Design review of the part built by this model. Coordinates are the model's own, in mm. A direction names the side the tool comes from. Coordinates: 2 decimals unless noted, no trailing zeros. Order: outer loops, then holes, each group sorted by start corner. A loop starts at its lowest first (then second) coordinate and runs counter-clockwise, first axis right, second up. Notation, with made-up numbers: M -39.75,18.25 L -19.75,18.25 A29 ccw -19.75,48.25 Z; hole C -31,-12.5 d11. An arc over 180 degrees is marked long. Use CSV: the item, a comma, the result in double quotes.
```python
from build123d import *

# Parameters (mm, degrees)
SKETCH_1_R          = 1.75
SKETCH_1_R_2        = 3
EXTRUDE_1_DEPTH     = 3
SKETCH_3_R          = 1.525
CUT_EXTRUDE_2_DEPTH = 10
SKETCH_5_R          = 1.55
CUT_EXTRUDE_3_DEPTH = 10


with BuildPart() as part:
    # 草图1 → 凸台-拉伸1 (new body)
    with BuildSketch(Plane.XY):
        Polygon((65, -25), (65, 75.163369284), (39.840227583, 104.667600302), (-39.840227583, 104.667600302), (-65, 75.163369284), (-65, -25), (-65, -35.332399698), (65, -35.332399698), align=None)
        with Locations((49.25, -15.332399698)):
            Circle(SKETCH_1_R, mode=Mode.SUBTRACT)
        with Locations((25.25, -15.332399698)):
            Circle(SKETCH_1_R, mode=Mode.SUBTRACT)
        with Locations((25.25, 15)):
            Circle(SKETCH_1_R, mode=Mode.SUBTRACT)
        with Locations((49.25, 15)):
            Circle(SKETCH_1_R, mode=Mode.SUBTRACT)
        with Locations(Location((-49.25, 15, 0), (0, 0, 180))):
            Circle(SKETCH_1_R, mode=Mode.SUBTRACT)
        with Locations(Location((-25.25, 15, 0), (0, 0, 180))):
            Circle(SKETCH_1_R, mode=Mode.SUBTRACT)
        with Locations(Location((-25.25, -15.332399698, 0), (0, 0, 180))):
            Circle(SKETCH_1_R, mode=Mode.SUBTRACT)
        with Locations(Location((-49.25, -15.332399698, 0), (0, 0, 180))):
            Circle(SKETCH_1_R, mode=Mode.SUBTRACT)
        with Locations((-17.5, 94.667600302)):
            Circle(SKETCH_1_R_2, mode=Mode.SUBTRACT)
        with Locations(Location((17.5, 94.667600302, 0), (0, 0, 180))):
            Circle(SKETCH_1_R_2, mode=Mode.SUBTRACT)
        with Locations((-17.5, 49.667600302)):
            Circle(SKETCH_1_R_2, mode=Mode.SUBTRACT)
        with Locations(Location((17.5, 49.667600302, 0), (0, 0, 180))):
            Circle(SKETCH_1_R_2, mode=Mode.SUBTRACT)
        with BuildLine():
            Line((-10, 39.667600302), (10, 39.667600302))
            ThreePointArc((10, 39.667600302), (11.5, 38.167600302), (10, 36.667600302))
            Line((10, 36.667600302), (-10, 36.667600302))
            ThreePointArc((-10, 36.667600302), (-11.5, 38.167600302), (-10, 39.667600302))
        make_face(mode=Mode.SUBTRACT)
        with BuildLine():
            Line((-10, -18.332399698), (10, -18.332399698))
            ThreePointArc((10, -18.332399698), (11.5, -19.832399698), (10, -21.332399698))
            Line((10, -21.332399698), (-10, -21.332399698))
            ThreePointArc((-10, -21.332399698), (-11.5, -19.832399698), (-10, -18.332399698))
        make_face(mode=Mode.SUBTRACT)
    extrude(amount=EXTRUDE_1_DEPTH)

    # 草图3 → 切除-拉伸2 (cut)
    with BuildSketch(Plane(origin=(0, 0, 0), x_dir=(-1, 0, 0), z_dir=(0, 0, -1))):
        with Locations((0, -25.832399698)):
            Circle(SKETCH_3_R)
        with BuildLine():
            Line((-18.52, -27.332399698), (-18.52, -24.332399698))
            ThreePointArc((-18.52, -24.332399698), (-17, -22.812399698), (-15.48, -24.332399698))
            Line((-15.48, -24.332399698), (-15.48, -27.332399698))
            ThreePointArc((-15.48, -27.332399698), (-17, -28.852399698), (-18.52, -27.332399698))
        make_face()
        with BuildLine():
            Line((18.52, -27.332399698), (18.52, -24.332399698))
            ThreePointArc((18.52, -24.332399698), (17, -22.812399698), (15.48, -24.332399698))
            Line((15.48, -24.332399698), (15.48, -27.332399698))
            ThreePointArc((15.48, -27.332399698), (17, -28.852399698), (18.52, -27.332399698))
        make_face()
    extrude(amount=-CUT_EXTRUDE_2_DEPTH, mode=Mode.SUBTRACT)

    # 草图5 → 切除-拉伸3 (cut)
    with BuildSketch(Plane.XY.offset(3)):
        with Locations((-47.5, 49.667600302)):
            Circle(SKETCH_5_R)
        with Locations((47.5, 49.667600302)):
            Circle(SKETCH_5_R)
        with Locations((-47.5, -25.332399698)):
            Circle(SKETCH_5_R)
        with Locations((47.5, -25.332399698)):
            Circle(SKETCH_5_R)
    extrude(amount=-CUT_EXTRUDE_3_DEPTH, mode=Mode.SUBTRACT)


solid = part.part
```
(1) Add section A-A on y = 15. State the section outline as (x, z) points.
The answers:
outline,"M -65,0 L -51,0 L -51,3 L -65,3 Z; M -47.5,0 L -27,0 L -27,3 L -47.5,3 Z; M -23.5,0 L 23.5,0 L 23.5,3 L -23.5,3 Z; M 27,0 L 47.5,0 L 47.5,3 L 27,3 Z; M 51,0 L 65,0 L 65,3 L 51,3 Z"
(2) Add section C-C on z = 2.2. Give the number of separate pieces and of enclosed holes in the cut face, and give its area (3 significant figures).
The answers:
separate pieces,"1"
enclosed holes,"21"
area,"17,100 mm2"
(3) For faces 4 (the face through (-15.48, -26, 1)), 5 (the face through (65, 19, 1)), list the 3-axis set-ups (+Z, -Z, +X, -X, +Y, -Y) from which the entire face can be reached by the end or side of a thin tool; tool diameter is ignored.
The answers:
face 4,"+Z, -Z"
face 5,"+Z, -Z, +X, +Y, -Y"
(4) Wall thickness on probe 1 along Y at (x, z) = (-25.5, 0.8); probe 2 along Y at (x, z) = (10, 1.1); probe 3 along Y at (x, z) = (17.5, 1.05): over which ranges is each line inside the solid? List them lowest first.
The answers:
probe 1,"y = -35.33 to -17.06, -13.6 to 13.27, 16.73 to 104.67"
probe 2,"y = -35.33 to -21.33, -18.33 to 36.67, 39.67 to 104.67"
probe 3,"y = -35.33 to -28.77, -22.9 to 46.67, 52.67 to 91.67, 97.67 to 104.67"
(5) Clearance check with a flat-ended pin moving along its axis: P1, Ø3, axis at x = -47.5, y = -25.33, coming from the -Z side. State where the tip first meets the part, or that it passes through.
The answers:
P1,"passes through"
(6) Add section D-D on x = 56.5. State the section outline as (y, z) points, and give its area (3 significant figures).
The answers:
outline,"M -35.33,0 L 85.13,0 L 85.13,3 L -35.33,3 Z"
area,"361 mm2"
(7) The part is to be moulded in two halves that separate along X. For faces 1 (the face through (0, -18.332, 1)), 2 (the face through (-65, 21, 1)), 3 (the face through (1, 104.668, 1)), say which applies: pulls with the +X half, pulls with the -X half, needs draft (parallel to the pull), parting line crosses it, or undercut.
The answers:
face 1,"undercut"
face 2,"pulls with the -X half"
face 3,"needs draft"
(8) Add section B-B on x = -54.5. State the section outline as (y, z) points, and give its area (3 significant figures).
The answers:
outline,"M -35.33,0 L 87.48,0 L 87.48,3 L -35.33,3 Z"
area,"368 mm2"
